Can you work these out from the model? Positions are in its coordinate system, mm. Coordinates: 2 decimals unless noted, no trailing zeros. Order: outer loops, then holes, each group sorted by start corner. A loop starts at its lowest first (then second) coordinate and runs counter-clockwise, first axis right, second up. Notation, with made-up numbers: (69.25, 20.5) - (76.25, 20.5) arc R32 ccw to (76.25, 49.5) - close; hole circle Ø3 at (9.5, 33). An arc over 180 degrees is marked (long way). Use a Markdown table: item, result. Add a question column.
(1) I want a section at A-A (y = -10.5). List the corners of the cut face in (x, z) for me, and give its area (3 significant figures).
(2) For pin 1 Ø6.5 at (x, y) = (0, 0) entering from +Z; pin 2 Ø10 at (y, z) = (-14.5, 7.5) entering from +X; pin 3 Ø10 at (x, z) = (2.5, 17) entering from -Y, each with a flat end and sliding along its axis, tell me the tip position at first contact or that it passes through.
(3) I want a section at D-D (x = 26). List the corners of the cut face in (y, z) for me, and give its area (3 significant figures).
(4) I want a section at B-B (y = 6). List the corners of the cut face in (x, z) for me, and give its area (3 significant figures).
(5) I want a section at C-C (z = 7.75). State how many separate pieces and enclosed holes the cut face has, and give its area (3 significant figures).
(6) If I drill on L1, parallel to Y at x = 0, z = 13; L2, parallel to X at y = 0.5, z = 18.25; L3, parallel to Y at x = 17, z = 16, over which ranges is the centre line in solid material (lowest first)? Write a range as [from, to].
(7) We'd pull the mould along X, two halves only. Please class faces 1 (the flat face through (7.73, -11.82, 9.13)), 2 (the flat face through (-8, 22, 20)), 3 (the flat face through (-3.22, 13.75, 9.13)), 4 (the cylindrical face through (31, 9.76, 9.86)): pulls with the +X half, pulls with the -X half, needs draft (parallel to the pull), parting line crosses it, or undercut.
```python
from build123d import *

# Parameters (mm, degrees)
CROQUIS1_R              = 32.5
SALIENTE_EXTRUIR1_DEPTH = 20
CROQUIS2_R              = 2
CORTAR_EXTRUIR1_DEPTH   = 20
CORTAR_EXTRUIR2_DEPTH   = 20
CROQUIS4_R              = 23
CORTAR_EXTRUIR3_DEPTH   = 2


with BuildPart() as part:
    # Croquis1 → Saliente-Extruir1 (new body)
    with BuildSketch(Plane.XY):
        Circle(CROQUIS1_R)
    extrude(amount=SALIENTE_EXTRUIR1_DEPTH)

    # Croquis2 → Cortar-Extruir1 (cut)
    with BuildSketch(Plane(origin=(0, 0, 0), x_dir=(-1, 0, 0), z_dir=(0, 0, -1))):
        Circle(CROQUIS2_R)
    extrude(amount=-CORTAR_EXTRUIR1_DEPTH, mode=Mode.SUBTRACT)

    # Croquis3 → Cortar-Extruir2 (cut)
    with BuildSketch(Plane.XY.offset(20)):
        with BuildLine():
            Line((1.140137938, 4.868273357), (5.244634516, 22.394057444))
            ThreePointArc((5.244634516, 22.394057444), (0, 23), (-5.244634516, 22.394057444))
            Line((-5.244634516, 22.394057444), (-1.140137938, 4.868273357))
            ThreePointArc((-1.140137938, 4.868273357), (0, 5), (1.140137938, 4.868273357))
        make_face()
        with BuildLine():
            Line((4.002662127, 2.996447213), (18.412245782, 13.78365718))
            ThreePointArc((18.412245782, 13.78365718), (14.784115023, 17.619022192), (10.376999529, 20.526029348))
            Line((10.376999529, 20.526029348), (2.255869463, 4.462180293))
            ThreePointArc((2.255869463, 4.462180293), (3.213938048, 3.830222216), (4.002662127, 2.996447213))
        make_face()
        with BuildLine():
            Line((4.992296221, -0.277449884), (22.964562618, -1.276269467))
            ThreePointArc((22.964562618, -1.276269467), (22.650578319, 3.993908086), (21.143120166, 9.053643998))
            Line((21.143120166, 9.053643998), (4.596330471, 1.968183478))
            ThreePointArc((4.596330471, 1.968183478), (4.924038765, 0.868240888), (4.992296221, -0.277449884))
        make_face()
        with BuildLine():
            Line((3.645979431, -3.421525097), (16.771505382, -15.739015446))
            ThreePointArc((16.771505382, -15.739015446), (19.918584287, -11.5), (22.016139898, -6.655041998))
            Line((22.016139898, -6.655041998), (4.786117369, -1.44674826))
            ThreePointArc((4.786117369, -1.44674826), (4.330127019, -2.5), (3.645979431, -3.421525097))
        make_face()
        with BuildLine():
            Line((0.593668344, -4.964630691), (2.730874383, -22.837301178))
            ThreePointArc((2.730874383, -22.837301178), (7.866463296, -21.612930278), (12.58756309, -19.249759881))
            Line((12.58756309, -19.249759881), (2.736426759, -4.184730409))
            ThreePointArc((2.736426759, -4.184730409), (1.710100717, -4.698463104), (0.593668344, -4.964630691))
        make_face()
        with BuildLine():
            Line((-2.736426759, -4.184730409), (-12.58756309, -19.249759881))
            ThreePointArc((-12.58756309, -19.249759881), (-7.866463296, -21.612930278), (-2.730874383, -22.837301178))
            Line((-2.730874383, -22.837301178), (-0.593668344, -4.964630691))
            ThreePointArc((-0.593668344, -4.964630691), (-1.710100717, -4.698463104), (-2.736426759, -4.184730409))
        make_face()
        with BuildLine():
            Line((-4.786117369, -1.44674826), (-22.016139898, -6.655041998))
            ThreePointArc((-22.016139898, -6.655041998), (-19.918584287, -11.5), (-16.771505382, -15.739015446))
            Line((-16.771505382, -15.739015446), (-3.645979431, -3.421525097))
            ThreePointArc((-3.645979431, -3.421525097), (-4.330127019, -2.5), (-4.786117369, -1.44674826))
        make_face()
        with BuildLine():
            Line((-4.596330471, 1.968183478), (-21.143120166, 9.053643998))
            ThreePointArc((-21.143120166, 9.053643998), (-22.650578319, 3.993908086), (-22.964562618, -1.276269467))
            Line((-22.964562618, -1.276269467), (-4.992296221, -0.277449884))
            ThreePointArc((-4.992296221, -0.277449884), (-4.924038765, 0.868240888), (-4.596330471, 1.968183478))
        make_face()
        with BuildLine():
            Line((-2.255869463, 4.462180293), (-10.376999529, 20.526029348))
            ThreePointArc((-10.376999529, 20.526029348), (-14.784115023, 17.619022192), (-18.412245782, 13.78365718))
            Line((-18.412245782, 13.78365718), (-4.002662127, 2.996447213))
            ThreePointArc((-4.002662127, 2.996447213), (-3.213938048, 3.830222216), (-2.255869463, 4.462180293))
        make_face()
    extrude(amount=-CORTAR_EXTRUIR2_DEPTH, mode=Mode.SUBTRACT)

    # Croquis4 → Cortar-Extruir3 (cut)
    with BuildSketch(Plane.XY.offset(20)):
        with Locations(Location((0, 0, 0), (0, 0, 356.819024652))):
            Circle(CROQUIS4_R)
    extrude(amount=-CORTAR_EXTRUIR3_DEPTH, mode=Mode.SUBTRACT)


solid = part.part
```
Answers follow:
| question | item | result |
|---|---|---|
| 1 | outline | (-30.76, 0) - (-20.46, 0) - (-20.46, 20) - (-30.76, 20) - close; (-11.19, 0) - (-6.87, 0) - (-6.87, 18) - (-11.19, 18) - close; (-1.26, 0) - (1.26, 0) - (1.26, 18) - (-1.26, 18) - close; (6.87, 0) - (11.19, 0) - (11.19, 18) - (6.87, 18) - close; (20.46, 0) - (30.76, 0) - (30.76, 20) - (20.46, 20) - close |
| 1 | area | 613 mm² |
| 2 | pin 1 | stops at z = 18 |
| 2 | pin 2 | stops at x = 31.08 |
| 2 | pin 3 | stops at y = -32.5 |
| 3 | outline | (-19.5, 0) - (19.5, 0) - (19.5, 20) - (-19.5, 20) - close |
| 3 | area | 780 mm² |
| 4 | outline | (-31.94, 0) - (-22.2, 0) - (-22.2, 20) - (-31.94, 20) - close; (-14.01, 0) - (-8.01, 0) - (-8.01, 18) - (-14.01, 18) - close; (-3.03, 0) - (-1.41, 0) - (-1.41, 18) - (-3.03, 18) - close; (1.41, 0) - (3.03, 0) - (3.03, 18) - (1.41, 18) - close; (8.01, 0) - (14.01, 0) - (14.01, 18) - (8.01, 18) - close; (22.2, 0) - (31.94, 0) - (31.94, 20) - (22.2, 20) - close |
| 4 | area | 664 mm² |
| 5 | separate pieces | 1 |
| 5 | enclosed holes | 10 |
| 5 | area | 2,260 mm² |
| 6 | L1 | y = [-32.5, -2], [2, 5], [23, 32.5] |
| 6 | L2 | x = [-32.5, -22.99], [22.99, 32.5] |
| 6 | L3 | y = [-27.7, -15.49], [-5.14, -0.94], [7.28, 12.73], [15.49, 27.7] |
| 7 | face 1 | undercut |
| 7 | face 2 | needs draft |
| 7 | face 3 | undercut |
| 7 | face 4 | parting line crosses it |
